Verification items for the finished model (mm, model axes). Face numbers are marked on the shaded views. Round coordinates to 2 decimals unless told otherwise and drop trailing zeros. Loops run counter-clockwise (first coordinate to the right, second up) from the corner with the lowest first, then second, coordinate; pieces in that order, holes last. Notation, with made-up numbers: (50.5, 1.25) -> (80.5, 1.25) arc R20 cw to (80.5, 29.25) -> close; hole circle Ø9 at (66.25, -38.75). An arc over 180 degrees is marked (long way). Use CSV: the item, a comma, the result in double quotes. Start each with the question number.
```python
from build123d import *

# Parameters (mm, degrees)
SKETCH1_R           = 37.973
SKETCH1_R_2         = 29.0322
BOSS_EXTRUDE1_DEPTH = 15.875
SKETCH3_R           = 39.624
SKETCH3_R_2         = 27.3304
BOSS_EXTRUDE2_DEPTH = 4.7625
SKETCH4_R           = 2.0193
CUT_EXTRUDE1_DEPTH  = 38.5445
CIRPATTERN2_COUNT   = 4
SKETCH5_R           = 2.0193
CUT_EXTRUDE2_DEPTH  = 52.2605
CIRPATTERN3_COUNT   = 4


with BuildPart() as part:
    # Sketch1 → Boss-Extrude1 (new body)
    with BuildSketch(Plane(origin=(0, 0, 0), x_dir=(1, 0, 0), z_dir=(0, 1, 0))):
        with Locations(Location((0, 0, 0), (0, 0, 270))):
            Circle(SKETCH1_R)
        with Locations(Location((0, 0, 0), (0, 0, 270))):
            Circle(SKETCH1_R_2, mode=Mode.SUBTRACT)
    extrude(amount=BOSS_EXTRUDE1_DEPTH)

    # Sketch3 → Boss-Extrude2 (add)
    with BuildSketch(Plane(origin=(0, 15.875, 0), x_dir=(1, 0, 0), z_dir=(0, 1, 0))):
        with Locations(Location((0, 0, 0), (0, 0, 90))):
            Circle(SKETCH3_R)
        with Locations(Location((0, 0, 0), (0, 0, 90))):
            Circle(SKETCH3_R_2, mode=Mode.SUBTRACT)
    extrude(amount=BOSS_EXTRUDE2_DEPTH)

    # Sketch4 → Cut-Extrude1 (cut)
    with BuildSketch(Plane(origin=(0, 20.6375, 0), x_dir=(1, 0, 0), z_dir=(0, 1, 0))):
        with Locations(Location((33.4772, 0, 0), (0, 0, 270))):
            Circle(SKETCH4_R)
    cut_extrude1 = extrude(amount=-CUT_EXTRUDE1_DEPTH, mode=Mode.SUBTRACT)

    # CirPattern2: Cut-Extrude1 ×4 about axis
    cirpattern2_axis = Axis((0, 0, 0), (0, 1, 0))
    for i in range(1, CIRPATTERN2_COUNT):
        add(cut_extrude1.rotate(cirpattern2_axis, i * 360 / CIRPATTERN2_COUNT), mode=Mode.SUBTRACT)

    # Sketch5 → Cut-Extrude2 (cut)
    with BuildSketch(Plane(origin=(0, 0, 0), x_dir=(-0.7071067811865477, 0, -0.7071067811865475), z_dir=(0.7071067811865475, 0, -0.7071067811865477))):
        with Locations((0, 7.9375)):
            Circle(SKETCH5_R)
    cut_extrude2 = extrude(amount=-CUT_EXTRUDE2_DEPTH, mode=Mode.SUBTRACT)

    # CirPattern3: Cut-Extrude2 ×4 about axis
    cirpattern3_axis = Axis((0, 15.875, 0), (0, -1, 0))
    for i in range(1, CIRPATTERN3_COUNT):
        add(cut_extrude2.rotate(cirpattern3_axis, i * 360 / CIRPATTERN3_COUNT), mode=Mode.SUBTRACT)


solid = part.part
```
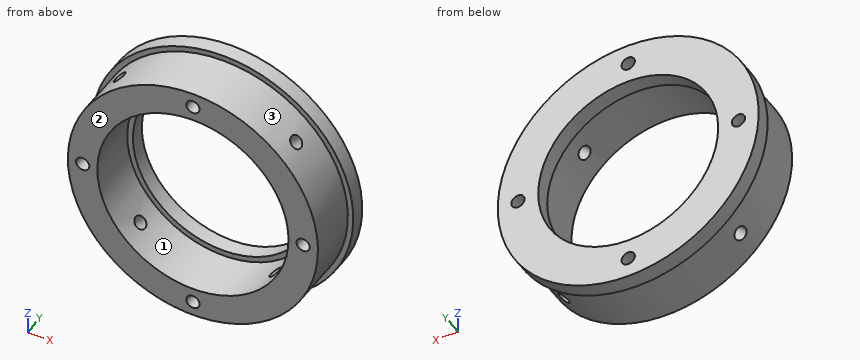
Q1. Cross-section at C-C (z = -18). Record the boundary of the cut face in (x, y) (1 decimal).
Q2. Cross-section at B-B (z = 0). Record the boundary of the cut face in (x, y) (1 decimal).
Q3. Cross-section at A-A (x = 0). Record the boundary of the cut face in (y, z) (1 decimal), and give its area (3 significant figures).
Q4. Depth check by flat-ended pin: pin 1 Ø1 at (y, z) = (12.5, -31.5) entering from +X; pin 2 Ø1.5 at (y, z) = (15, -6) entering from +X; pin 3 Ø3.5 at (x, z) = (-33.48, 0) entering from -Y; pin 4 Ø2 at (x, y) = (11, 5.5) entering from +Z. Enter the tip coordinate at first touch or a pass-through.
Q5. Release check for a two-part mould opening along X. For the marked faces 1, 2 and 3 record: +X half, -X half, draft (parallel to the pull), parting line (faces both ways), or undercut.
Q6. Cross-section at D-D (y = 17.25). Record the boundary of the cut face in (x, z).
Q7. Thickness scan on L1, parallel to X at y = 17.3, z = 0; L2, parallel to X at y = 15.25, z = 0; L3, parallel to Z at x = -1, y = 10.5. Record the ranges inside material, lowest first. Write a range as from..to.
Answer list:
1,outline,"(-35.3, 15.9) -> (-33.4, 15.9) -> (-33.4, 0) -> (-22.8, 0) -> (-22.8, 15.9) -> (-20.6, 15.9) -> (-20.6, 20.6) -> (-35.3, 20.6) -> close; (20.6, 15.9) -> (22.8, 15.9) -> (22.8, 0) -> (33.4, 0) -> (33.4, 15.9) -> (35.3, 15.9) -> (35.3, 20.6) -> (20.6, 20.6) -> close"
2,outline,"(-39.6, 15.9) -> (-38, 15.9) -> (-38, 0) -> (-35.5, 0) -> (-35.5, 20.6) -> (-39.6, 20.6) -> close; (-31.5, 0) -> (-29, 0) -> (-29, 15.9) -> (-27.3, 15.9) -> (-27.3, 20.6) -> (-31.5, 20.6) -> close; (27.3, 15.9) -> (29, 15.9) -> (29, 0) -> (31.5, 0) -> (31.5, 20.6) -> (27.3, 20.6) -> close; (35.5, 0) -> (38, 0) -> (38, 15.9) -> (39.6, 15.9) -> (39.6, 20.6) -> (35.5, 20.6) -> close"
3,outline,"(0, -38) -> (15.9, -38) -> (15.9, -39.6) -> (20.6, -39.6) -> (20.6, -35.5) -> (0, -35.5) -> close; (0, -31.5) -> (20.6, -31.5) -> (20.6, -27.3) -> (15.9, -27.3) -> (15.9, -29) -> (0, -29) -> close; (0, 29) -> (15.9, 29) -> (15.9, 27.3) -> (20.6, 27.3) -> (20.6, 31.5) -> (0, 31.5) -> close; (0, 35.5) -> (20.6, 35.5) -> (20.6, 39.6) -> (15.9, 39.6) -> (15.9, 38) -> (0, 38) -> close"
3,area,"234 mm2"
4,pin 1,"stops at x = 21.93"
4,pin 2,"stops at x = 37.61"
4,pin 3,"passes through"
4,pin 4,"stops at z = 36.63"
5,face 1,"undercut"
5,face 2,"draft"
5,face 3,"parting line"
6,outline,"circle Ø79.25 at (0, 0); hole circle Ø4.04 at (-33.48, 0); hole circle Ø54.66 at (0, 0); hole circle Ø4.04 at (0, -33.48); hole circle Ø4.04 at (0, 33.48); hole circle Ø4.04 at (33.48, 0)"
7,L1,"x = -39.62..-35.5, -31.46..-27.33, 27.33..31.46, 35.5..39.62"
7,L2,"x = -37.97..-35.5, -31.46..-29.03, 29.03..31.46, 35.5..37.97"
7,L3,"z = -37.96..-35.23, -31.72..-29.01, 29.01..31.72, 35.23..37.96"
